Can you work these out from the drawing? Everything is in mm from the part's minimum corner. A direction names the side the tool comes from. Round coordinates to 2 decimals unless told otherwise and drop trailing zeros. Order: outer loops, then holes, each group sorted by start corner. A loop starts at its lowest first (then second) coordinate and runs counter-clockwise, first axis right, second up. Notation, with made-up numbers: (22, 57.25) -> (38, 57.25) arc R28 cw to (38, 87.25) -> close; hole circle Ø5 at (89.5, -24). An arc over 180 degrees is marked (long way). One line per item, written item: value.
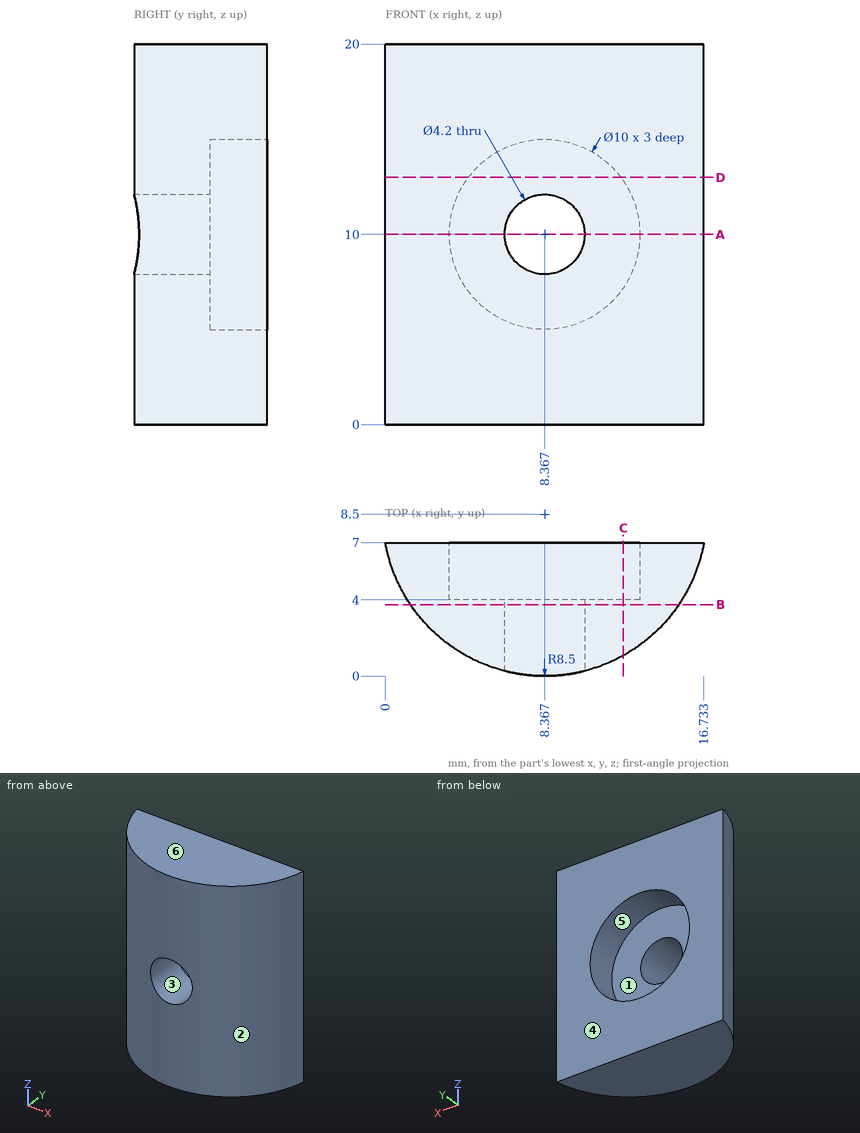
Q1. I want a section at D-D on z = 13. List the corners of the cut face in (x, y) for me.
Answers below:
outline: (0, 7) arc R8.5 ccw to (16.73, 7) -> (12.37, 7) -> (12.37, 4) -> (4.37, 4) -> (4.37, 7) -> close
Q2. I want a section at C-C on x = 12.5. List the corners of the cut face in (y, z) for me.
Answers below:
outline: (1.07, 0) -> (7, 0) -> (7, 7.19) -> (4, 7.19) -> (4, 12.81) -> (7, 12.81) -> (7, 20) -> (1.07, 20) -> close
Q3. I want a section at A-A on z = 10. List the corners of the cut face in (x, y) for me.
Answers below:
outline: (0, 7) arc R8.5 ccw to (6.27, 0.26) -> (6.27, 4) -> (3.37, 4) -> (3.37, 7) -> close; (10.47, 0.26) arc R8.5 ccw to (16.73, 7) -> (13.37, 7) -> (13.37, 4) -> (10.47, 4) -> close
Q4. Please list where these lines run through material, in increasing order: line 1 along X through (y, z) = (3, 11) (1 decimal); line 2 along X through (y, z) = (1.5, 10.5) (1 decimal); line 3 along Z through (x, y) = (10, 5.75) (1 decimal).
Answers below:
line 1: 1.9 to 6.5, 10.2 to 14.8
line 2: 3.5 to 6.3, 10.4 to 13.2
line 3: 0 to 5.3, 14.7 to 20
Q5. Will these pins go through, and if not, where does the flat tip stop? pin 1 Ø5 at (x, z) = (2, 2) entering from -Y; pin 2 Ø9 at (x, z) = (8.37, 10) entering from +Y; pin 3 Ø1.5 at (y, z) = (4.5, 7) entering from -X.
Answers below:
pin 1: y = 0.93
pin 2: y = 4
pin 3: x = 0.51
Q6. We'd pull the mould along X, two halves only. Please class the marked faces 1, 2, 3 and 4: released by +X, released by -X, zero draft, split by the parting line, or undercut.
Answers below:
face 1: undercut
face 2: split by the parting line
face 3: undercut
face 4: zero draft
Q7. I want a section at B-B on y = 3.75. List the corners of the cut face in (x, z) for me (1 decimal).
Answers below:
outline: (1.3, 0) -> (15.4, 0) -> (15.4, 20) -> (1.3, 20) -> close; hole circle Ø4.2 at (8.4, 10)
Q8. On a 3-axis mill with a long thin cutter (end or side, diameter ignored), from which of +Z, -Z, +X, -X, +Y, -Y can I reach the whole of each face in a straight line? I mean the marked faces 5 and 6. Say none if no direction works.
Answers below:
face 5: +Y
face 6: +Z, +X, -X, +Y, -Y
